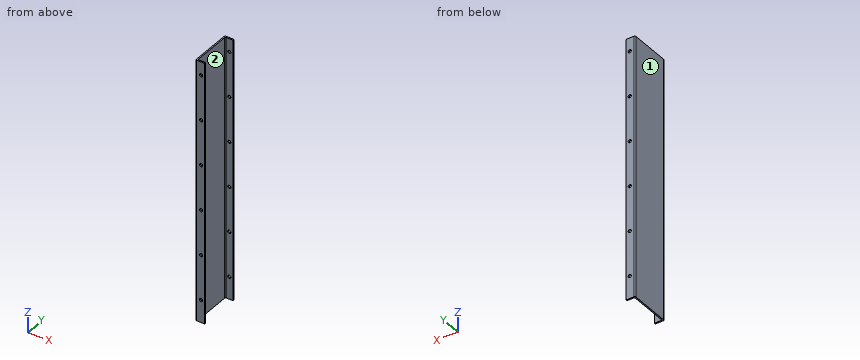
```python
from build123d import *

# Parameters (mm, degrees)
SKETCH1_W           = 1.5
SKETCH1_H           = 43.5
BOSS_EXTRUDE1_DEPTH = 289.77
FILLET1_R           = 1
SKETCH3_R           = 1.75
CUT_EXTRUDE1_DEPTH  = 246.38


with BuildPart() as part:
    # Sketch1 → Boss-Extrude1 (new body)
    with BuildSketch(Plane.XY):
        Rectangle(SKETCH1_W, SKETCH1_H)
        Polygon((-0.75, 23.25), (-0.75, 21.75), (0.75, 21.75), (9.25, 21.75), (9.25, 23.25), align=None)
        Polygon((0.75, -21.75), (-0.75, -21.75), (-0.75, -23.25), (9.25, -23.25), (9.25, -21.75), align=None)
    extrude(amount=BOSS_EXTRUDE1_DEPTH)

    # Fillet1
    fillet1_edges = [part.edges().sort_by_distance(p)[0] for p in [
        (0.75, -21.75, 144.885),
        (-0.75, -23.25, 144.885),
        (-0.75, 23.25, 144.885),
        (0.75, 21.75, 144.885),
    ]]
    fillet(fillet1_edges, radius=FILLET1_R)

    # Sketch3 → Cut-Extrude1 (cut)
    with BuildSketch(Plane(origin=(0, -23.25, 0), x_dir=(-1, 0, 0), z_dir=(0, -1, 0))):
        with Locations((-5.25, -25)):
            Circle(SKETCH3_R)
        with Locations((-5.25, -75)):
            Circle(SKETCH3_R)
        with Locations((-5.25, -125)):
            Circle(SKETCH3_R)
        with Locations((-5.25, -175)):
            Circle(SKETCH3_R)
        with Locations((-5.25, -225)):
            Circle(SKETCH3_R)
        with Locations((-5.25, -275)):
            Circle(SKETCH3_R)
    extrude(amount=-CUT_EXTRUDE1_DEPTH, mode=Mode.SUBTRACT)


solid = part.part
```
For this review, take the finished solid that the model builds, in its own axes (mm). Face numbers are marked on the shaded views. Give positions to 0.01 mm unless a question says otherwise; leave off trailing zeros. Write each loop counter-clockwise with the first axis right and the second up, starting at its lowest first coordinate (ties: lowest second). Pieces come first, ordered by that corner, then holes.
Item 1: Take a section at C-C (y = 18). Give the boundary of the cut face in (x, z).
Item 2: Wall thickness on probe 1 along Y at (x, z) = (6.25, 162.5); probe 2 along X at (y, z) = (-22.3, 175): over which ranges is each line inside the solid? List them lowest first.
Item 3: Insertion check: P1, Ø5, axis at y = -16.5, z = 41.5, coming from the +X side; P2, Ø2, axis at x = 5.25, z = 75, coming from the -Y side. Each pin has a flat end and moves straight along its axis. Give the tip position at first contact, or say it passes through.
Item 4: Take a section at B-B (x = 5.25). Give the number of separate pieces and of enclosed holes in the cut face, and give its area (3 significant figures).
Item 5: Take a section at A-A (z = 106). Give the boundary of the cut face in (x, y).
Item 6: The part is to be moulded in two halves that separate along Y. For the marked faces 1 and 2, say which applies: +Y half, -Y half, draft (parallel to the pull), parting line (faces both ways), or undercut.
Established:
1. outline: (-0.75, 0) - (0.75, 0) - (0.75, 289.77) - (-0.75, 289.77) - close
2. probe 1: y = -23.25 to -21.75, 21.75 to 23.25
2. probe 2: x = -0.75 to 3.5, 7 to 9.25
3. P1: stops at x = 0.75
3. P2: passes through
4. separate pieces: 14
4. enclosed holes: 0
4. area: 806 mm2
5. outline: (-0.75, -22.25) arc R1 ccw to (0.25, -23.25) - (9.25, -23.25) - (9.25, -21.75) - (1.75, -21.75) arc R1 cw to (0.75, -20.75) - (0.75, 20.75) arc R1 cw to (1.75, 21.75) - (9.25, 21.75) - (9.25, 23.25) - (0.25, 23.25) arc R1 ccw to (-0.75, 22.25) - close
6. face 1: draft
6. face 2: undercut
